Geometry: final body of the model. Coordinates: model frame, mm. Give positions to 0.01 mm unless a question says otherwise; leave off trailing zeros. Order: outer loops, then holes, each group sorted by start corner. A loop starts at its lowest first (then second) coordinate and runs counter-clockwise, first axis right, second up. Notation, with made-up numbers: (76, 22) -> (89, 22) arc R20 ccw to (89, 44) -> close; hole circle Ø11 at (85, 4). An arc over 180 degrees is marked (long way). One line per question, with ' | ' between items. Start each with the question number.
(1) Section C-C (z = -32.5). Return loops of the section in (x, y), then the cut area to 3 significant figures.
(2) Ray query, L1, parallel to Z at x = -0.5, y = 6; L2, parallel to Z at x = -14, y = 17; L3, parallel to Z at x = -37.5, y = 4.75. Return the intervals inside material, ascending.
(3) First-contact query: pin 1 Ø1 at (x, y) = (-29, 17) entering from +Z; pin 2 Ø1.5 at (x, z) = (37.5, -40) entering from -Y; pin 3 Ø1 at (x, y) = (-43.5, 15.5) entering from -Z. Flat tips, straight axial feed; report the tip coordinate or a pass-through.
(4) Section A-A (y = 6.5). State how many separate pieces and enclosed holes the cut face has, then the cut area to 3 significant figures.
(5) Mould query, pull axis Z, two halves, no side actions, for faces 1 (the face through (31.4, 10.14, -11.054)), 2 (the face through (62.464, 12.325, -8.201)), 3 (the face through (-43.59, 9.86, -41.23)). Classes: +Z half, -Z half, draft (parallel to the pull), parting line (faces both ways), or undercut.
(6) Section B-B (x = -34). Return loops of the section in (y, z).
```python
from build123d import *

# Parameters (mm, degrees)
SKETCH1_R           = 63
BOSS_EXTRUDE1_DEPTH = 25
SKETCH2_R           = 60
CUT_EXTRUDE2_DEPTH  = 20
SKETCH3_R           = 7.5
BOSS_EXTRUDE2_DEPTH = 20
EXTRUDE_THIN3_DEPTH = 20


with BuildPart() as part:
    # Sketch1 → Boss-Extrude1 (new body)
    with BuildSketch(Plane(origin=(0, 0, 0), x_dir=(1, 0, 0), z_dir=(0, 1, 0))):
        with Locations(Location((0, 0, 0), (0, 0, 270))):
            Circle(SKETCH1_R)
    extrude(amount=BOSS_EXTRUDE1_DEPTH)

    # Sketch2 → Cut-Extrude2 (cut)
    with BuildSketch(Plane.XZ):
        with Locations(Location((0, 0, 0), (0, 0, 270))):
            Circle(SKETCH2_R)
    extrude(amount=-CUT_EXTRUDE2_DEPTH, mode=Mode.SUBTRACT)

    # Sketch3 → Boss-Extrude2 (add)
    with BuildSketch(Plane.XZ.offset(-20)):
        with Locations(Location((0, 0, 0), (0, 0, 270))):
            Circle(SKETCH3_R)
    extrude(amount=BOSS_EXTRUDE2_DEPTH)

    # Sketch4 → Extrude-Thin3 (add, through all)
    with BuildSketch(Plane.XZ.offset(-20)):
        Polygon((-23.273288682, 57.13837857), (23.273288682, -57.13837857), (21.421043823, -57.892824713), (-25.125533541, 56.383932427), align=None)
        Polygon((23.946234705, 56.8596352), (-23.946234705, -56.8596352), (-25.789443589, -56.083374284), (22.103025822, 57.635896117), align=None)
        Polygon((57.13837857, 23.273288682), (-57.13837857, -23.273288682), (-57.892824713, -21.421043823), (56.383932427, 25.125533541), align=None)
        Polygon((56.8596352, -23.946234705), (-56.8596352, 23.946234705), (-56.083374284, 25.789443589), (57.635896117, -22.103025822), align=None)
    extrude(amount=EXTRUDE_THIN3_DEPTH)


solid = part.part
```
Response:
1) outline: (-53.97, 0) -> (-50.44, 0) -> (-50.44, 20) -> (-15.86, 20) -> (-15.86, 0) -> (-13.69, 0) -> (-13.69, 20) -> (11.08, 20) -> (11.08, 0) -> (13.24, 0) -> (13.24, 20) -> (50.44, 20) -> (50.44, 0) -> (53.97, 0) -> (53.97, 25) -> (-53.97, 25) -> close | area: 768 mm^2
2) L1: z = -63 to -60, -7.48 to 7.48, 60 to 63 | L2: z = -61.42 to -58.34, -33.24 to -28.09, -5.7 to -3.54, 5.9 to 8.07, 29.07 to 34.37, 58.34 to 61.42 | L3: z = -50.62 to -46.84, -15.27 to -13.11, 15.79 to 17.96, 46.84 to 50.62
3) pin 1: stops at z = 56.18 | pin 2: stops at y = 20 | pin 3: stops at z = -46.04
4) separate pieces: 1 | enclosed holes: 8 | area: 2,180 mm^2
5) face 1: undercut | face 2: parting line | face 3: undercut
6) outline: (0, -53.04) -> (25, -53.04) -> (25, 53.04) -> (0, 53.04) -> (0, 49.44) -> (20, 49.44) -> (20, 16.49) -> (0, 16.49) -> (0, 14.32) -> (20, 14.32) -> (20, -11.69) -> (0, -11.69) -> (0, -13.85) -> (20, -13.85) -> (20, -49.44) -> (0, -49.44) -> close
